Verification items for the finished model (mm, model axes). A direction names the side the tool comes from. Give positions to 0.01 mm unless a question says otherwise; leave off trailing zeros. Loops run counter-clockwise (first coordinate to the right, second up) from the corner with the lowest first, then second, coordinate; pieces in that order, holes last. Notation, with made-up numbers: M 29.5,-1 L 35.5,-1 A20 cw 35.5,23 Z; hole C 34.5,80 d2. An arc over 180 degrees is marked long. Put each result on its own line as item: value. Start each with the question number.
from build123d import *

# Parameters (mm, degrees)
SKETCH1_W              = 9.525
SKETCH1_H              = 33.3375
COMBINE1_START         = -168.91
COMBINE1_OUTLINE_R     = 5.55625
COMBINE1_DEPTH         = 20.91
COMBINE1_START_2       = -152.4
COMBINE1_2_OUTLINE_R   = 6.35
COMBINE1_2_OUTLINE_R_2 = 5.55625
COMBINE1_2_DEPTH       = 4.4
COMBINE1_START_3       = -166.890966931
COMBINE1_3_OUTLINE_R   = 1.0795
COMBINE1_3_DEPTH       = 2.743466931
COMBINE1_4_OUTLINE_R   = 1.0795
COMBINE1_4_OUTLINE_R_2 = 6.35
COMBINE1_4_DEPTH       = 10.107803
COMBINE1_5_OUTLINE_R   = 6.35
COMBINE1_5_OUTLINE_R_2 = 5.55625
COMBINE1_5_DEPTH       = 4.7625
COMBINE1_START_4       = -164.1475
COMBINE1_6_OUTLINE_R   = 1.0795
COMBINE1_6_DEPTH       = 1.8256249
COMBINE1_START_5       = 4.7625
COMBINE1_7_OUTLINE_R   = 3.571875
COMBINE1_7_DEPTH       = 4.7625
COMBINE1_START_6       = -11
COMBINE1_8_OUTLINE_R   = 1.7272
COMBINE1_8_DEPTH       = 15.7625
COMBINE1_START_7       = 0.793749963
COMBINE1_9_OUTLINE_R   = 2.1844
COMBINE1_9_OUTLINE_R_2 = 1.7272
COMBINE1_9_DEPTH       = 3.968750037
COMBINE1_START_8       = -33.3375
COMBINE1_10_OUTLINE_R  = 1.1303
COMBINE1_10_DEPTH      = 3.297532088


with BuildPart() as part:
    # Sketch1 → Revolve1 (revolve)
    with BuildSketch(Plane(origin=(0, 0, 0), x_dir=(1, 0, 0), z_dir=(0, 1, 0))):
        with Locations((-153.9875, 16.66875)):
            Rectangle(SKETCH1_W, SKETCH1_H)
    revolve(axis=Axis((-158.75, 0, 0), (0, 0, -1)))

    # Combine1: read off the stored shape, not the designer's step
    # Combine1 outline → Combine1 (cut)
    with BuildSketch(Plane.YZ.offset(COMBINE1_START)):
        with BuildLine():
            Line((0.79375, 0), (-0.79375, 0))
            Line((-0.79375, 0), (-0.793749936, -8.394440501))
            ThreePointArc((-0.793749936, -8.394440501), (-1e-08, -17.052925), (0.793749959, -8.394440505))
            Line((0.793749959, -8.394440505), (0.79375, 0))
        make_face()
        with Locations((0, -24.5999)):
            Circle(COMBINE1_OUTLINE_R)
    extrude(amount=COMBINE1_DEPTH, mode=Mode.SUBTRACT)

    # Combine1 2 outline → Combine1 2 (cut)
    with BuildSketch(Plane.YZ.offset(COMBINE1_START_2)):
        with Locations((0, -24.5999)):
            Circle(COMBINE1_2_OUTLINE_R)
        with Locations((0, -24.5999)):
            Circle(COMBINE1_2_OUTLINE_R_2, mode=Mode.SUBTRACT)
    extrude(amount=COMBINE1_2_DEPTH, mode=Mode.SUBTRACT)

    # Combine1 3 outline → Combine1 3 (cut)
    with BuildSketch(Plane.YZ.offset(COMBINE1_START_3)):
        with Locations((7.14375, -19.8374)):
            Circle(COMBINE1_3_OUTLINE_R)
        with Locations((-7.14375, -29.3624)):
            Circle(COMBINE1_3_OUTLINE_R)
    extrude(amount=COMBINE1_3_DEPTH, mode=Mode.SUBTRACT)

    # Combine1 4 outline → Combine1 4 (add)
    with BuildSketch(Plane.YZ.offset(COMBINE1_START)):
        with BuildLine():
            Line((-9.525, 0), (-9.525, -33.3375))
            Line((-9.525, -33.3375), (9.525, -33.3375))
            Line((9.525, -33.3375), (9.525, 0))
            Line((9.525, 0), (0.79375, 0))
            Line((0.79375, 0), (0.793749959, -8.394440505))
            ThreePointArc((0.793749959, -8.394440505), (-1e-08, -17.052925), (-0.793749936, -8.394440501))
            Line((-0.793749936, -8.394440501), (-0.79375, 0))
            Line((-0.79375, 0), (-9.525, 0))
        make_face()
        with Locations((-7.14375, -29.3624)):
            Circle(COMBINE1_4_OUTLINE_R, mode=Mode.SUBTRACT)
        with Locations((0, -24.5999)):
            Circle(COMBINE1_4_OUTLINE_R_2, mode=Mode.SUBTRACT)
        with Locations((7.14375, -19.8374)):
            Circle(COMBINE1_4_OUTLINE_R, mode=Mode.SUBTRACT)
    extrude(amount=COMBINE1_4_DEPTH)

    # Combine1 5 outline → Combine1 5 (add)
    with BuildSketch(Plane.YZ.offset(COMBINE1_START)):
        with Locations((0, -24.5999)):
            Circle(COMBINE1_5_OUTLINE_R)
        with Locations((0, -24.5999)):
            Circle(COMBINE1_5_OUTLINE_R_2, mode=Mode.SUBTRACT)
    extrude(amount=COMBINE1_5_DEPTH)

    # Combine1 6 outline → Combine1 6 (add)
    with BuildSketch(Plane.YZ.offset(COMBINE1_START_4)):
        with Locations((7.14375, -19.8374)):
            Circle(COMBINE1_6_OUTLINE_R)
        with Locations((-7.14375, -29.3624)):
            Circle(COMBINE1_6_OUTLINE_R)
    extrude(amount=COMBINE1_6_DEPTH)

    # Combine1 7 outline → Combine1 7 (cut)
    with BuildSketch(Plane(origin=(0, 0, 0), x_dir=(1, 0, 0), z_dir=(0, 1, 0)).offset(COMBINE1_START_5)):
        with Locations((-158.75, 4.9911)):
            Circle(COMBINE1_7_OUTLINE_R)
    extrude(amount=COMBINE1_7_DEPTH, mode=Mode.SUBTRACT)

    # Combine1 8 outline → Combine1 8 (cut)
    with BuildSketch(Plane(origin=(0, 0, 0), x_dir=(1, 0, 0), z_dir=(0, 1, 0)).offset(COMBINE1_START_6)):
        with Locations((-158.75, 4.9911)):
            Circle(COMBINE1_8_OUTLINE_R)
    extrude(amount=COMBINE1_8_DEPTH, mode=Mode.SUBTRACT)

    # Combine1 9 outline → Combine1 9 (cut)
    with BuildSketch(Plane(origin=(0, 0, 0), x_dir=(1, 0, 0), z_dir=(0, 1, 0)).offset(COMBINE1_START_7)):
        with Locations((-158.75, 4.9911)):
            Circle(COMBINE1_9_OUTLINE_R)
        with Locations((-158.75, 4.9911)):
            Circle(COMBINE1_9_OUTLINE_R_2, mode=Mode.SUBTRACT)
    extrude(amount=COMBINE1_9_DEPTH, mode=Mode.SUBTRACT)

    # Combine1 10 outline → Combine1 10 (cut)
    with BuildSketch(Plane.XY.offset(COMBINE1_START_8)):
        with Locations((-158.75, 0)):
            Circle(COMBINE1_10_OUTLINE_R)
    extrude(amount=COMBINE1_10_DEPTH, mode=Mode.SUBTRACT)


solid = part.part
Q1. Cross-section at D-D, the plane y = -3. Record the boundary of the cut face in (x, z), then the cut area to 3 significant figures.
Q2. Release check for a two-part mould opening along Z. For faces 6 (the face through (-168.91, -4, -16)), 7 (the face through (-151.19, -5.04, -28.46)), 8 (the face through (-159, 5, 0)) record: pulls with the +Z half, pulls with the -Z half, needs draft (parallel to the pull), parting line crosses it, or undercut.
Q3. Set-up check for faces 1 (the face through (-162.32, 7.11, -5.15)), 2 (the face through (-164.148, 7, -20)), 3 (the face through (-152.4, 4, -29)), 4 (the face through (-159.88, 0.05, -31.71)), 5 (the face through (-159, -0.794, -3)): record each of +Z, -Z, +X, -X, +Y, -Y from which the full face is reachable in a straight line by a thin tool's end or side.
Q4. Cross-section at B-B, the plane x = -152. Record the boundary of the cut face in (y, z).
Q5. Scan lines: L1, parallel to Y at x = -168, z = -5 (3 decimals); L2, parallel to Y at x = -162, z = -6 (1 decimal); L3, parallel to Z at x = -166.75, y = 1.75. Record each from-to range of solid material in increasing order.
Q6. Go/stop test with flat-tipped pins: pin 1 (6 mm diameter, centred on y = 7.5, z = -28, fed in from +X); pin 2 (0.6 mm diameter, centred on y = 6.5, z = -19.5, fed in from -X); pin 3 (4 mm diameter, centred on x = -152.5, y = 1, fed in from +Z); pin 4 (3.5 mm diameter, centred on y = -7.14, z = -29.36, fed in from +X). Record where each tip stops, or that it passes through.
Q7. Cross-section at A-A, the plane y = 0. Record the boundary of the cut face in (x, z) (1 decimal), then the cut area to 3 significant figures.
Ans:
1. outline: M -168.91,-33.34 L -149.71,-33.34 L -149.71,-30.2 L -152.4,-30.2 L -152.4,-29.28 L -168.91,-29.28 Z; M -168.91,-19.92 L -152.4,-19.92 L -152.4,-19 L -149.71,-19 L -149.71,-15.86 L -168.91,-15.86 Z; M -168.91,-9.52 L -149.71,-9.52 L -149.71,0 L -168.91,0 Z; hole C -158.75,-4.99 d3.45
1. area: 324 mm^2
2. face 6: needs draft
2. face 7: undercut
2. face 8: pulls with the +Z half
3. face 1: +Y
3. face 2: -X
3. face 3: +X
3. face 4: -Z
3. face 5: +Z, +X, -X
4. outline: M -6.72,-33.34 L 6.72,-33.34 L 6.72,0 L 0.79,0 L 0.79,-8.39 A4.37 cw long -0.79,-8.39 L -0.79,0 L -6.72,0 Z; hole C 0,-24.6 d12.7
5. L1: y = -9.525 to -0.794, 0.794 to 9.525
5. L2: y = -9.5 to -0.8, 0.8 to 4.8
5. L3: z = -33.34 to -29.87, -19.33 to -16.69, -8.69 to 0
6. pin 1: stops at x = -150.44
6. pin 2: stops at x = -164.15
6. pin 3: stops at z = 0
6. pin 4: stops at x = -150.9
7. outline: M -168.9,-33.3 L -159.9,-33.3 L -159.9,-30.2 L -168.9,-30.2 Z; M -168.9,-19 L -152.4,-19 L -152.4,-18.2 L -149.2,-18.2 L -149.2,-17.1 L -168.9,-17.1 Z; M -157.6,-33.3 L -149.2,-33.3 L -149.2,-30.9 L -152.4,-30.9 L -152.4,-30.2 L -157.6,-30.2 Z
7. area: 89.6 mm^2
